```python
from build123d import *

# Parameters (mm, degrees)
SKETCH1_R           = 75
BOSS_EXTRUDE1_DEPTH = 25
SKETCH2_W           = 15
SKETCH2_H           = 30
BOSS_EXTRUDE2_DEPTH = 25
FILLET1_R           = 3
FILLET2_R           = 5
SKETCH3_R           = 1.25
BOSS_EXTRUDE3_DEPTH = 10
SKETCH4_R           = 1.25
BOSS_EXTRUDE4_DEPTH = 10
SKETCH5_R           = 1.25
BOSS_EXTRUDE5_DEPTH = 10
SKETCH6_R           = 1.25
BOSS_EXTRUDE6_DEPTH = 10
SKETCH7_R           = 1.25
BOSS_EXTRUDE7_DEPTH = 10
SKETCH8_R           = 1.25
BOSS_EXTRUDE8_DEPTH = 10
CHAMFER1_SIZE       = 10


with BuildPart() as part:
    # Sketch1 → Boss-Extrude1 (new body)
    with BuildSketch(Plane(origin=(0, 0, 0), x_dir=(1, 0, 0), z_dir=(0, 1, 0))):
        Circle(SKETCH1_R)
    extrude(amount=BOSS_EXTRUDE1_DEPTH)

    # Sketch2 → Boss-Extrude2 (add)
    with BuildSketch(Plane(origin=(0, 25, 0), x_dir=(1, 0, 0), z_dir=(0, 1, 0))):
        Polygon((-64.371778265, -28.504809472), (-56.871778265, -41.495190528), (-30.891016151, -26.495190528), (-38.391016151, -13.504809472), align=None)
        with Locations((0, 55)):
            Rectangle(SKETCH2_W, SKETCH2_H)
        Polygon((64.371778265, -28.504809472), (56.871778265, -41.495190528), (30.891016151, -26.495190528), (38.391016151, -13.504809472), align=None)
    extrude(amount=BOSS_EXTRUDE2_DEPTH)

    # Fillet1
    fillet1_edges = [part.edges().sort_by_distance(p)[0] for p in [
        (-7.5, 25, -55),
        (0, 25, -40),
        (7.5, 25, -55),
        (0, 25, -70),
        (51.381397208, 25, 21.004809472),
        (34.641016151, 25, 20),
        (43.881397208, 25, 33.995190528),
        (60.621778265, 25, 35),
        (-51.381397208, 25, 21.004809472),
        (-60.621778265, 25, 35),
        (-43.881397208, 25, 33.995190528),
        (-34.641016151, 25, 20),
    ]]
    fillet(fillet1_edges, radius=FILLET1_R)

    # Fillet2
    fillet2_edges = [part.edges().sort_by_distance(p)[0] for p in [
        (-7.5, 50, -55),
        (7.5, 50, -55),
        (51.381397208, 50, 21.004809472),
        (43.881397208, 50, 33.995190528),
        (-51.381397208, 50, 21.004809472),
        (-43.881397208, 50, 33.995190528),
    ]]
    fillet(fillet2_edges, radius=FILLET2_R)

    # Sketch3 → Boss-Extrude3 (add)
    with BuildSketch(Plane(origin=(60.621778265, 0, 35), x_dir=(0.5, 0, -0.866025404), z_dir=(0.866025404, 0, 0.5))):
        with Locations((0, 45)):
            Circle(SKETCH3_R)
    extrude(amount=BOSS_EXTRUDE3_DEPTH)

    # Sketch4 → Boss-Extrude4 (add)
    with BuildSketch(Plane(origin=(34.641016151, 0, 20), x_dir=(-0.5, 0, 0.866025404), z_dir=(-0.866025404, 0, -0.5))):
        with Locations((0, 45)):
            Circle(SKETCH4_R)
    extrude(amount=BOSS_EXTRUDE4_DEPTH)

    # Sketch5 → Boss-Extrude5 (add)
    with BuildSketch(Plane(origin=(0, 0, -70), x_dir=(-1, 0, 0), z_dir=(0, 0, -1))):
        with Locations((0, 45)):
            Circle(SKETCH5_R)
    extrude(amount=BOSS_EXTRUDE5_DEPTH)

    # Sketch6 → Boss-Extrude6 (add)
    with BuildSketch(Plane.XY.offset(-40)):
        with Locations((0, 45)):
            Circle(SKETCH6_R)
    extrude(amount=BOSS_EXTRUDE6_DEPTH)

    # Sketch7 → Boss-Extrude7 (add)
    with BuildSketch(Plane(origin=(-60.621778265, 0, 35), x_dir=(0.5, 0, 0.866025404), z_dir=(-0.866025404, 0, 0.5))):
        with Locations((0, 45)):
            Circle(SKETCH7_R)
    extrude(amount=BOSS_EXTRUDE7_DEPTH)

    # Sketch8 → Boss-Extrude8 (add)
    with BuildSketch(Plane(origin=(-34.641016151, 0, 20), x_dir=(-0.5, 0, -0.866025404), z_dir=(0.866025404, 0, -0.5))):
        with Locations((0, 45)):
            Circle(SKETCH8_R)
    extrude(amount=BOSS_EXTRUDE8_DEPTH)

    # Chamfer1
    chamfer1_edges = [part.edges().sort_by_distance(p)[0] for p in [
        (-75, 0, 0),
    ]]
    chamfer(chamfer1_edges, length=CHAMFER1_SIZE)


solid = part.part
```
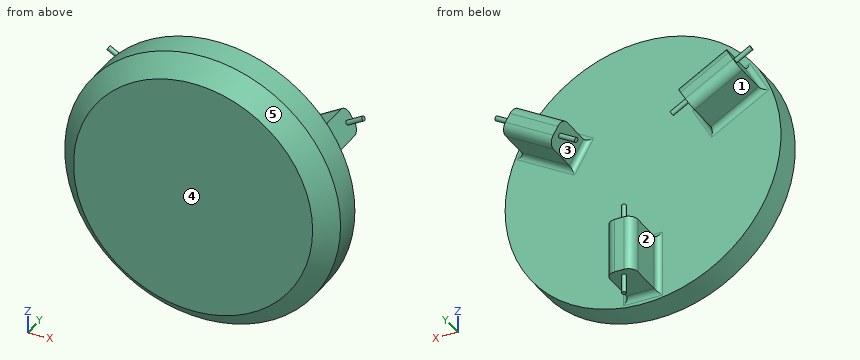
Here's how the part is built. I have some questions about the finished solid (model axes, mm). Face numbers are marked on the shaded views. A direction names the side the tool comes from. Coordinates: 2 decimals unless noted, no trailing zeros. Loops run counter-clockwise (first coordinate to the right, second up) from the corner with the lowest first, then second, coordinate; pieces in that order, holes last. Notation, with made-up numbers: (46, 57) - (61, 57) arc R20 ccw to (61, 67) - close; hole circle Ø8 at (32, 20). An arc over 180 degrees is marked (long way). Return JSON: item names as keys, results as strings. Group by question number.
Item 1: We'd pull the mould along X, two halves only. Please class the marked faces 3, 4 and 5: +X half, -X half, draft (parallel to the pull), parting line (faces both ways), or undercut.
Item 2: If we section it at C-C on y = 13.5: Write out the boundary of the cut face in (x, z), and give its area (3 significant figures).
Item 3: Will these pins go through, and if not, where does the flat tip stop? P1, Ø1, axis at x = 6, y = 36, coming from the +Z side; P2, Ø10, axis at x = -0.5, z = 9.5, coming from the -Y side; P3, Ø3, axis at x = -50.5, y = 9.5, coming from the +Z side; P4, Ø13.5, axis at y = 40, z = -59.5, coming from the +X side.
Item 4: I need wall thicknesses on line 1 (X direction, y = 44.5, z = -44); line 2 (Y direction, x = 33.5, z = -21); line 3 (Z direction, x = 5, y = 28). Which ranges of each line are inside material? Lowest first, please. Write a range as from..to.
Item 5: If we section it at A-A on y = 30: Write out the boundary of the cut face in (x, z), and give its area (3 significant figures).
Item 6: If we section it at B-B on z = 0: Write out the boundary of the cut face in (x, y), and give its area (3 significant figures).
Item 7: On a 3-axis mill with a long thin cutter (end or side, diameter ignored), from which of +Z, -Z, +X, -X, +Y, -Y can I reach the whole of each face in a straight line? I mean the marked faces 1 and 2. Say none if no direction works.
Calculated:
{
 "1": {"face 3": "undercut", "face 4": "draft", "face 5": "parting line"},
 "2": {"outline": "circle Ø150 at (0, 0)", "area": "17,700 mm^2"},
 "3": {"P1": "stops at z = -40", "P2": "stops at y = 0", "P3": "stops at z = 56.71", "P4": "stops at x = 7.5"},
 "4": {"line 1": "x = -7.5..7.5", "line 2": "y = 0..25", "line 3": "z = -70..-40"},
 "5": {"outline": "(-64.37, 28.5) - (-38.39, 13.5) - (-30.89, 26.5) - (-56.87, 41.5) - close; (-7.5, -70) - (7.5, -70) - (7.5, -40) - (-7.5, -40) - close; (30.89, 26.5) - (38.39, 13.5) - (64.37, 28.5) - (56.87, 41.5) - close", "area": "1,350 mm^2"},
 "6": {"outline": "(-75, 10) - (-65, 0) - (65, 0) - (75, 10) - (75, 25) - (-75, 25) - close", "area": "3,650 mm^2"},
 "7": {"face 1": "-Z, -X, +Y", "face 2": "+Z, -Z, -X, +Y"}
}
